from build123d import *

# Parameters (mm, degrees)
ESQUISSE1_W             = 236
ESQUISSE1_H             = 78
BOSS_EXTRU_1_DEPTH      = 3
ENL_V_MAT_EXTRU_1_REACH = 126.314
ESQUISSE2_R             = 2
ESQUISSE3_W             = 236
ESQUISSE3_H             = 6
BOSS_EXTRU_2_DEPTH      = 3
ENL_V_MAT_EXTRU_2_REACH = 128.325


with BuildPart() as part:
    # Esquisse1 → Boss.-Extru.1 (new body)
    with BuildSketch(Plane.XY):
        Rectangle(ESQUISSE1_W, ESQUISSE1_H)
    extrude(amount=BOSS_EXTRU_1_DEPTH)

    # Esquisse2 → Enl_v. mat.-Extru.1 (cut, up to next)
    with BuildSketch(Plane.XY.offset(3), mode=Mode.PRIVATE) as enl_v_mat_extru_1_sk1:
        with Locations((9, -26)):
            Circle(ESQUISSE2_R)
    enl_v_mat_extru_1_tool1 = extrude(enl_v_mat_extru_1_sk1.sketch, amount=-ENL_V_MAT_EXTRU_1_REACH, mode=Mode.PRIVATE) & part.part
    # Esquisse2 → Enl_v. mat.-Extru.1 (cut, up to next)
    with BuildSketch(Plane.XY.offset(3), mode=Mode.PRIVATE) as enl_v_mat_extru_1_sk2:
        with Locations((-9, -26)):
            Circle(ESQUISSE2_R)
    enl_v_mat_extru_1_tool2 = extrude(enl_v_mat_extru_1_sk2.sketch, amount=-ENL_V_MAT_EXTRU_1_REACH, mode=Mode.PRIVATE) & part.part
    enl_v_mat_extru_1_1 = enl_v_mat_extru_1_tool1.solids().sort_by_distance((9, -26, 3))[0]
    add(enl_v_mat_extru_1_1, mode=Mode.SUBTRACT)
    enl_v_mat_extru_1_2 = enl_v_mat_extru_1_tool2.solids().sort_by_distance((-9, -26, 3))[0]
    add(enl_v_mat_extru_1_2, mode=Mode.SUBTRACT)
    enl_v_mat_extru_1 = enl_v_mat_extru_1_1 + enl_v_mat_extru_1_2  # Enl_v. mat.-Extru.1 as one shape, for the pattern or mirror that repeats it

    # Sym_trie1: Enl_v. mat.-Extru.1 across plane
    add(enl_v_mat_extru_1.mirror(Plane.ZX), mode=Mode.SUBTRACT)

    # Esquisse3 → Boss.-Extru.2 (add)
    with BuildSketch(Plane.XY.offset(3)):
        with Locations((0, -42)):
            Rectangle(ESQUISSE3_W, ESQUISSE3_H)
    extrude(amount=-BOSS_EXTRU_2_DEPTH)

    # Esquisse4 → Enl_v. mat.-Extru.2 (cut, up to next)
    with BuildSketch(Plane.XY.offset(3), mode=Mode.PRIVATE) as enl_v_mat_extru_2_sk1:
        Polygon((34, -36), (34, -3), (43, 6), (77, 6), (86, -3), (86, -36), align=None)
    enl_v_mat_extru_2_tool1 = extrude(enl_v_mat_extru_2_sk1.sketch, amount=-ENL_V_MAT_EXTRU_2_REACH, mode=Mode.PRIVATE) & part.part
    # Esquisse4 → Enl_v. mat.-Extru.2 (cut, up to next)
    with BuildSketch(Plane.XY.offset(3), mode=Mode.PRIVATE) as enl_v_mat_extru_2_sk2:
        Polygon((-86, -3), (-77, 6), (-43, 6), (-34, -3), (-34, -36), (-86, -36), align=None)
    enl_v_mat_extru_2_tool2 = extrude(enl_v_mat_extru_2_sk2.sketch, amount=-ENL_V_MAT_EXTRU_2_REACH, mode=Mode.PRIVATE) & part.part
    add(enl_v_mat_extru_2_tool1.solids().sort_by_distance((60, -15.693295, 3))[0], mode=Mode.SUBTRACT)
    add(enl_v_mat_extru_2_tool2.solids().sort_by_distance((-60, -15.693295, 3))[0], mode=Mode.SUBTRACT)


solid = part.part
Geometry: final body of the model. Coordinates: model frame, mm. A direction names the side the tool comes from. Round coordinates to 2 decimals unless told otherwise and drop trailing zeros. Write each loop counter-clockwise with the first axis right and the second up, starting at its lowest first coordinate (ties: lowest second). Pieces come first, ordered by that corner, then holes. Notation, with made-up numbers: M 11,25 L 63,25 A37 cw 63,62 Z; hole C -33.75,6.5 d8. An arc over 180 degrees is marked long. Write item = value, one per line.
Item 1: Pin query (flat end, axial travel): P1, Ø3, axis at x = 9, y = 26, coming from the -Z side. Return the tip coordinate at first contact, or that it passes through.
Findings:
P1 = through
Item 2: Material intervals for line 1 along Y through (x, z) = (9, 1.5); line 2 along X through (y, z) = (26, 1.4); line 3 along X through (y, z) = (-28.5, 0.2), sorted ascending. Write a range as [from, to].
Findings:
line_1 = [-45, -28], [-24, 24], [28, 39]
line_2 = [-118, -11], [-7, 7], [11, 118]
line_3 = [-118, -86], [-34, 34], [86, 118]
Item 3: Section query D-D on x = -80. Return loops of the section in (y, z).
Findings:
outline = M -45,0 L -36,0 L -36,3 L -45,3 Z; M 3,0 L 39,0 L 39,3 L 3,3 Z
Item 4: Access query for faces 1 (the face through (-82, 1, 2)), 2 (the face through (-2, -2, 3)). Directions: +Z, -Z, +X, -X, +Y, -Y. A direction counts if a zero-diameter tool reaches every point of the face in a straight line with its end or side. Return the directions, or none.
Findings:
face_1 = +Z, -Z
face_2 = +Z, +X, -X, +Y, -Y
Item 5: Section query A-A on x = 71.5. Return loops of the section in (y, z).
Findings:
outline = M -45,0 L -36,0 L -36,3 L -45,3 Z; M 6,0 L 39,0 L 39,3 L 6,3 Z
Item 6: Section query C-C on y = -10. Return loops of the section in (x, z).
Findings:
outline = M -118,0 L -86,0 L -86,3 L -118,3 Z; M -34,0 L 34,0 L 34,3 L -34,3 Z; M 86,0 L 118,0 L 118,3 L 86,3 Z
Item 7: Section query B-B on z = 1.2. Return loops of the section in (x, y).
Findings:
outline = M -118,-45 L 118,-45 L 118,39 L -118,39 Z; hole M -86,-36 L -34,-36 L -34,-3 L -43,6 L -77,6 L -86,-3 Z; hole C -9,-26 d4; hole C -9,26 d4; hole C 9,-26 d4; hole C 9,26 d4; hole M 34,-36 L 86,-36 L 86,-3 L 77,6 L 43,6 L 34,-3 Z
